Work out the finished part from the listing and answer in its coordinate system (mm). A direction names the side the tool comes from. Round coordinates to 2 decimals unless told otherwise and drop trailing zeros. Order: outer loops, then holes, each group sorted by start corner. A loop starts at its lowest first (then second) coordinate and runs counter-clockwise, first axis right, second up. Notation, with made-up numbers: (62.25, -18) - (85.25, -18) arc R15 ccw to (85.25, -3) - close; hole circle Ø8 at (1, 40.25). An arc over 180 degrees is marked (long way). Use one line per item in the form item = value. Start each with the question number.
Q1. The part is cut by section A-A on z = 8.5. Determine the outline of the cut face in (x, y).
Q2. Given P1, Ø2.5, axis at x = 45.1, y = 6, coming from the -Z side; P2, Ø3, axis at x = 50, y = 18.5, coming from the -Z side; P3, Ø2.5, axis at x = 7, y = 17, coming from the -Z side, each flat-ended and moving along its own axis, determine where each tip first touches the part or whether it passes through.
Q3. Find the intervals of material crossed by line 1 (X direction, y = 76, z = 1.4); line 2 (Y direction, x = 6, z = 3.45); line 3 (Y direction, x = 45.1, z = 2.7), in increasing order. Write a range as [from, to].
Q4. The part is cut by section C-C on x = 18.5. Determine the outline of the cut face in (y, z), plus the area to 3 significant figures.
Q5. For a pull along Z with two mould halves and no side action, classify faces 6 (the flat face through (25, 79.5, 14)), 7 (the cylindrical face through (42.338, 73.176, 2.465)), 8 (the flat face through (6, 4, 5)), 9 (the flat face through (1, 41, 0)) as +Z half, -Z half, draft (parallel to the pull), parting line (faces both ways), or undercut.
Q6. The part is cut by section D-D on y = 19. Determine the outline of the cut face in (x, z), plus the area to 3 significant figures.
Q7. The part is cut by section B-B on y = 69. Determine the outline of the cut face in (x, z).
Q8. Which of the six approach directions +Z, -Z, +X, -X, +Y, -Y give full straight-line access (tool end or side, diameter ignored) to faces 1 (the cylindrical face through (5.686, 74.584, 2.465)), 2 (the flat face through (25, 0, 15)), 3 (the flat face through (25, 82, 15)), 4 (the flat face through (7, 9.376, 6)), 5 (the flat face through (6, 11.376, 2))?
from build123d import *

# Parameters (mm, degrees)
SKETCH1_W           = 51.1
SKETCH1_H           = 82
SKETCH1_R           = 1.45
BOSS_EXTRUDE1_DEPTH = 5
BOSS_EXTRUDE2_START = 5
SKETCH2_W           = 51.1
SKETCH2_H           = 82
SKETCH2_W_2         = 46.1
SKETCH2_H_2         = 77
BOSS_EXTRUDE2_DEPTH = 23
SKETCH4_W           = 2
SKETCH4_H           = 82
BOSS_EXTRUDE3_DEPTH = 51.1
SKETCH5_W           = 2.5
SKETCH5_H           = 18.7
CUT_EXTRUDE1_DEPTH  = 6
BOSS_EXTRUDE4_START = 5
SKETCH6_W           = 8.1
SKETCH6_H           = 18.7
BOSS_EXTRUDE4_DEPTH = 2
SKETCH7_W           = 8.1
SKETCH7_H           = 2
BOSS_EXTRUDE5_DEPTH = 7


with BuildPart() as part:
    # Sketch1 → Boss-Extrude1 (new body)
    with BuildSketch(Plane.XY):
        with Locations((25.55, 41)):
            Rectangle(SKETCH1_W, SKETCH1_H)
        with Locations((6, 76)):
            Circle(SKETCH1_R, mode=Mode.SUBTRACT)
        with Locations((45.1, 76)):
            Circle(SKETCH1_R, mode=Mode.SUBTRACT)
        with Locations((45.1, 6)):
            Circle(SKETCH1_R, mode=Mode.SUBTRACT)
        with Locations((6, 6)):
            Circle(SKETCH1_R, mode=Mode.SUBTRACT)
        with BuildLine():
            Line((6, 72.05), (2.5, 72.05))
            Line((2.5, 72.05), (2.5, 9.95))
            Line((2.5, 9.95), (6, 9.95))
            ThreePointArc((6, 9.95), (8.793071786, 8.793071786), (9.95, 6))
            Line((9.95, 6), (9.95, 2.5))
            Line((9.95, 2.5), (41.15, 2.5))
            Line((41.15, 2.5), (41.15, 6))
            ThreePointArc((41.15, 6), (42.306928214, 8.793071786), (45.1, 9.95))
            Line((45.1, 9.95), (48.6, 9.95))
            Line((48.6, 9.95), (48.6, 72.05))
            Line((48.6, 72.05), (45.1, 72.05))
            ThreePointArc((45.1, 72.05), (42.306928214, 73.206928214), (41.15, 76))
            Line((41.15, 76), (41.15, 79.5))
            Line((41.15, 79.5), (9.95, 79.5))
            Line((9.95, 79.5), (9.95, 76))
            ThreePointArc((9.95, 76), (8.793071786, 73.206928214), (6, 72.05))
        make_face(mode=Mode.SUBTRACT)
    extrude(amount=BOSS_EXTRUDE1_DEPTH)

    # Sketch2 → Boss-Extrude2 (add)
    with BuildSketch(Plane.XY.offset(BOSS_EXTRUDE2_START)):
        with Locations((25.55, 41)):
            Rectangle(SKETCH2_W, SKETCH2_H)
        with Locations((25.55, 41)):
            Rectangle(SKETCH2_W_2, SKETCH2_H_2, mode=Mode.SUBTRACT)
    extrude(amount=BOSS_EXTRUDE2_DEPTH)

    # Sketch4 → Boss-Extrude3 (add)
    with BuildSketch(Plane(origin=(0, 0, 0), x_dir=(0, 0, -1), z_dir=(1, 0, 0))):
        with Locations((-29, 41)):
            Rectangle(SKETCH4_W, SKETCH4_H)
    extrude(amount=BOSS_EXTRUDE3_DEPTH)

    # Sketch5 → Cut-Extrude1 (cut)
    with BuildSketch(Plane.XY):
        with Locations((49.85, 20.726044427)):
            Rectangle(SKETCH5_W, SKETCH5_H)
    extrude(amount=CUT_EXTRUDE1_DEPTH, mode=Mode.SUBTRACT)

    # Sketch6 → Boss-Extrude4 (add)
    with BuildSketch(Plane.XY.offset(BOSS_EXTRUDE4_START)):
        with Locations((6.55, 20.726044427)):
            Rectangle(SKETCH6_W, SKETCH6_H)
    extrude(amount=BOSS_EXTRUDE4_DEPTH)

    # Sketch7 → Boss-Extrude5 (add)
    with BuildSketch(Plane.XY):
        with Locations((6.55, 31.076044427)):
            Rectangle(SKETCH7_W, SKETCH7_H)
        with Locations((6.55, 10.376044427)):
            Rectangle(SKETCH7_W, SKETCH7_H)
    extrude(amount=BOSS_EXTRUDE5_DEPTH)


solid = part.part
Found:
q1.outline = (0, 0) - (51.1, 0) - (51.1, 82) - (0, 82) - close; hole (2.5, 2.5) - (48.6, 2.5) - (48.6, 79.5) - (2.5, 79.5) - close
q2.P1 = 28
q2.P2 = 6
q2.P3 = 5
q3.line_1 = [0, 4.55], [7.45, 9.95], [41.15, 43.65], [46.55, 51.1]
q3.line_2 = [0, 4.55], [7.45, 11.38], [30.08, 32.08], [72.05, 74.55], [77.45, 82]
q3.line_3 = [0, 4.55], [7.45, 9.95], [72.05, 74.55], [77.45, 82]
q4.outline = (0, 0) - (2.5, 0) - (2.5, 28) - (79.5, 28) - (79.5, 0) - (82, 0) - (82, 30) - (0, 30) - close
q4.area = 304 mm²
q5.face_6 = undercut
q5.face_7 = draft
q5.face_8 = undercut
q5.face_9 = -Z half
q6.outline = (0, 0) - (2.5, 0) - (2.5, 5) - (10.6, 5) - (10.6, 7) - (2.5, 7) - (2.5, 28) - (48.6, 28) - (48.6, 6) - (51.1, 6) - (51.1, 30) - (0, 30) - close
q6.area = 243 mm²
q7.outline = (0, 0) - (2.5, 0) - (2.5, 28) - (48.6, 28) - (48.6, 0) - (51.1, 0) - (51.1, 30) - (0, 30) - close
q8.face_1 = -Z
q8.face_2 = +Z, -Z, +X, -X, -Y
q8.face_3 = +Z, -Z, +X, -X, +Y
q8.face_4 = none
q8.face_5 = -Z, +X
